Design review of the part built by this model. Coordinates are the model's own, in mm. Give positions to 0.01 mm unless a question says otherwise; leave off trailing zeros. Loops run counter-clockwise (first coordinate to the right, second up) from the corner with the lowest first, then second, coordinate; pieces in that order, holes last.
from build123d import *

# Parameters (mm, degrees)
ESBO_O1_R                                  = 4.7625
RESSALTO_EXTRUS_O1_DEPTH                   = 12
CHANFRO1_SIZE                              = 0.5
CHANFRO1_SIZE2                             = 1.866025404
BROCA_DE_ROSQUEAR_PARA_TARRAXA_DE_5_16_1_D = 6.5278


with BuildPart() as part:
    # Esboço1 → Ressalto-extrusão1 (new body)
    with BuildSketch(Plane.XY):
        Circle(ESBO_O1_R)
    extrude(amount=RESSALTO_EXTRUS_O1_DEPTH)

    # Chanfro1
    chanfro1_edges = [part.edges().sort_by_distance(p)[0] for p in [
        (-4.7625, 0, 0),
    ]]
    chanfro1_side = [part.faces().sort_by_distance(p)[0] for p in [
        (0, 0, 0),
    ]]
    chamfer(chanfro1_edges, length=CHANFRO1_SIZE, length2=CHANFRO1_SIZE2, reference=chanfro1_side[0])

    # Broca de rosquear para tarraxa de 5/16-181 (through all)
    with Locations(Plane(origin=(0, 0, 0), x_dir=(-1, 0, 0), z_dir=(0, 0, -1))):
        with Locations((0, 0)):
            Hole(BROCA_DE_ROSQUEAR_PARA_TARRAXA_DE_5_16_1_D / 2)


solid = part.part
Q1. Insertion check: pin 1 (5 mm diameter, centred on x = 1.5, z = 10.5, fed in from -Y); pin 2 (3 mm diameter, centred on x = 2, z = 10.5, fed in from -Y). Each pin has a flat end and moves straight along its axis. Give the tip position at first contact, or say it passes through.
Results:
pin 1: stops at y = -4.76
pin 2: stops at y = -4.74
Q2. Take a section at D-D (z = 1). Give the boundary of the cut face in (x, y), plus the area to 3 significant figures.
Results:
outline: circle Ø9.06 at (0, 0); hole circle Ø6.53 at (0, 0)
area: 31.0 mm2
Q3. Wall thickness on line 1 (Y direction, x = 0, z = 4.25); line 2 (X direction, y = 0.25, z = 8.25); line 3 (Y direction, x = 1.5, z = 2): over which ranges is each line inside the solid? List them lowest first.
Results:
line 1: y = -4.76 to -3.26, 3.26 to 4.76
line 2: x = -4.76 to -3.25, 3.25 to 4.76
line 3: y = -4.52 to -2.9, 2.9 to 4.52
Q4. Take a section at A-A (y = 0). Give the boundary of the cut face in (x, z).
Results:
outline: (-4.76, 1.87) - (-4.26, 0) - (-3.26, 0) - (-3.26, 12) - (-4.76, 12) - close; (3.26, 0) - (4.26, 0) - (4.76, 1.87) - (4.76, 12) - (3.26, 12) - close
Q5. Take a section at C-C (z = 2.5). Give the boundary of the cut face in (x, y) (1 decimal), plus the area to 3 significant figures.
Results:
outline: circle Ø9.5 at (0, 0); hole circle Ø6.5 at (0, 0)
area: 37.8 mm2
Q6. Draft analysis for pull direction Y (two halves, no side actions). For faces 1 (the face through (-3.78, -2.9, 6.86)), 2 (the face through (-0.708, -3.186, 6.084)), 3 (the face through (2, -3, 0)), state which applies: pulls with the +Y half, pulls with the -Y half, needs draft (parallel to the pull), parting line crosses it, or undercut.
Results:
face 1: parting line crosses it
face 2: undercut
face 3: needs draft
